Answer from the drawing. Dimensions are ordinates in mm from the lowest x, y and z of the part. A direction names the side the tool comes from. Give positions to 0.01 mm unless a question says otherwise; leave off trailing zeros. Loops run counter-clockwise (first coordinate to the right, second up) from the corner with the lowest first, then second, coordinate; pieces in that order, holes last. Notation, with made-up numbers: (35, 32) -> (49, 32) arc R23 cw to (49, 53) -> close; hole circle Ø10 at (72, -22). An arc over 180 degrees is marked (long way). Return JSON: item names as keys, results as strings. Group by question number.
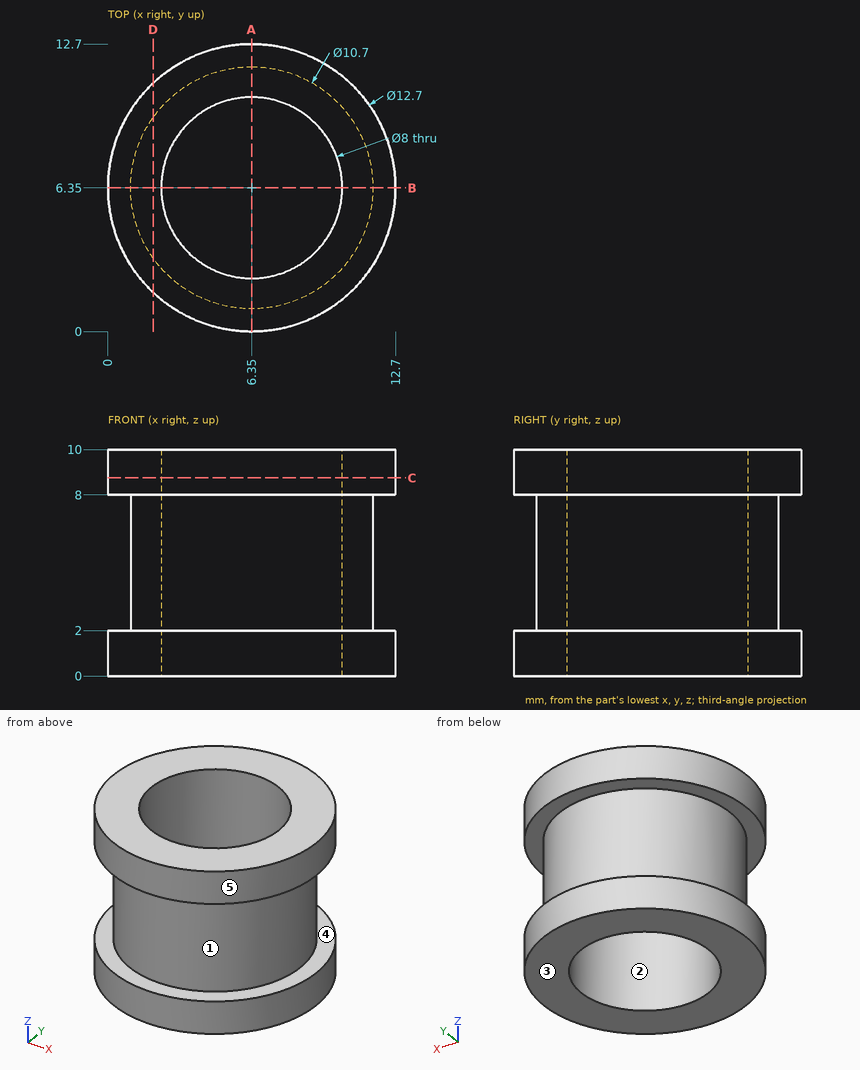
1. Which of the six approach directions +Z, -Z, +X, -X, +Y, -Y give full straight-line access (tool end or side, diameter ignored) to the marked faces 4 and 5?
2. Section D-D on x = 2 is taken. Determine the outline of the cut face in (y, z).
3. Flat-ended cylindrical pins translate along their axes: pin 1 Ø4 at (x, z) = (2.5, 6.5) entering from -Y; pin 2 Ø5 at (y, z) = (1.5, 5.5) entering from -X; pin 3 Ø5 at (y, z) = (10, 5) entering from +X. Find the tip coordinate at first contact, or state that the pin passes through.
4. Determine the mould class of the marked faces 1, 2 and 3 for opening direction X: pulls with the +X half, pulls with the -X half, needs draft (parallel to the pull), parting line crosses it, or undercut.
5. Straight lines are drawn through the part: line 1 (Z direction, x = 12.25, y = 4.75); line 2 (Y direction, x = 6.5, z = 4.75); line 3 (X direction, y = 7.25, z = 5). For each, find the intervals that lie inside material, in ascending order. Write a range as from..to.
6. Section C-C on z = 8.75 is taken. Determine the outline of the cut face in (x, y), then the cut area to 3 significant figures.
7. Section A-A on x = 6.35 is taken. Determine the outline of the cut face in (y, z), then the cut area to 3 significant figures.
Completed:
{
 "1": {"face 4": "none", "face 5": "+Z, -Z"},
 "2": {"outline": "(1.72, 0) -> (10.98, 0) -> (10.98, 2) -> (9.46, 2) -> (9.46, 8) -> (10.98, 8) -> (10.98, 10) -> (1.72, 10) -> (1.72, 8) -> (3.24, 8) -> (3.24, 2) -> (1.72, 2) -> close"},
 "3": {"pin 1": "stops at y = 0.52", "pin 2": "stops at x = 1.54", "pin 3": "stops at x = 11.57"},
 "4": {"face 1": "parting line crosses it", "face 2": "undercut", "face 3": "needs draft"},
 "5": {"line 1": "z = 0..2, 8..10", "line 2": "y = 1..2.35, 10.35..11.7", "line 3": "x = 1.08..2.45, 10.25..11.62"},
 "6": {"outline": "circle Ø12.7 at (6.35, 6.35); hole circle Ø8 at (6.35, 6.35)", "area": "76.4 mm²"},
 "7": {"outline": "(0, 0) -> (2.35, 0) -> (2.35, 10) -> (0, 10) -> (0, 8) -> (1, 8) -> (1, 2) -> (0, 2) -> close; (10.35, 0) -> (12.7, 0) -> (12.7, 2) -> (11.7, 2) -> (11.7, 8) -> (12.7, 8) -> (12.7, 10) -> (10.35, 10) -> close", "area": "35.0 mm²"}
}
